Work out the finished part from the listing and answer in its coordinate system (mm). A direction names the side the tool comes from. Round coordinates to 2 decimals unless told otherwise and drop trailing zeros. Write each loop counter-clockwise with the first axis right and the second up, starting at its lowest first coordinate (ties: lowest second). Pieces come first, ordered by that corner, then holes. Notation, with made-up numbers: (-29.5, -38.75) - (25.5, -38.75) arc R32 ccw to (25.5, -3.75) - close; hole circle Ø1 at (-6, 57). An arc over 180 degrees is marked (long way). Answer as a JSON object with one key per item and string values.
```python
from build123d import *

# Parameters (mm, degrees)
BOSS_EXTRUDE1_DEPTH = 33
BOSS_EXTRUDE2_DEPTH = 33
FILLET1_R           = 4
FILLET3_R           = 4
SKETCH3_R           = 1.35
CUT_EXTRUDE1_DEPTH  = 10
SKETCH4_R           = 2.5
CUT_EXTRUDE2_DEPTH  = 1
FILLET4_R           = 4


with BuildPart() as part:
    # Sketch1 → Boss-Extrude1 (new body)
    with BuildSketch(Plane.XY):
        with BuildLine():
            Line((-9.736529156, -5.734980384), (-6, -5.734980384))
            ThreePointArc((-6, -5.734980384), (0, 8.3), (6, -5.734980384))
            Line((6, -5.734980384), (9.736529156, -5.734980384))
            ThreePointArc((9.736529156, -5.734980384), (0, 11.3), (-9.736529156, -5.734980384))
        make_face()
    extrude(amount=BOSS_EXTRUDE1_DEPTH)

    # Sketch2 → Boss-Extrude2 (add)
    with BuildSketch(Plane(origin=(0, 0, 0), x_dir=(-1, 0, 0), z_dir=(0, 0, -1))):
        with BuildLine():
            Line((-10.464206022, 4.265019616), (-18.736529156, 4.265019616))
            Line((-18.736529156, 4.265019616), (-18.736529156, -10.734980384))
            Line((-18.736529156, -10.734980384), (-38.736529156, -10.734980384))
            Line((-38.736529156, -10.734980384), (-38.736529156, -13.734980384))
            Line((-38.736529156, -13.734980384), (-13.736529156, -13.734980384))
            Line((-13.736529156, -13.734980384), (-13.736529156, -5.734980384))
            Line((-13.736529156, -5.734980384), (-9.736529156, -5.734980384))
            ThreePointArc((-9.736529156, -5.734980384), (-11.270200772, -0.820106438), (-10.464206022, 4.265019616))
        make_face()
    extrude(amount=-BOSS_EXTRUDE2_DEPTH)

    # Fillet1
    fillet1_edges = [part.edges().sort_by_distance(p)[0] for p in [
        (18.736529156, 4.265019616, 16.5),
        (10.464206022, 4.265019616, 16.5),
    ]]
    fillet(fillet1_edges, radius=FILLET1_R)

    # Fillet3
    fillet3_edges = [part.edges().sort_by_distance(p)[0] for p in [
        (13.736529156, -5.734980384, 16.5),
    ]]
    fillet(fillet3_edges, radius=FILLET3_R)

    # Sketch3 → Cut-Extrude1 (cut)
    with BuildSketch(Plane(origin=(0, -10.734980384, 0), x_dir=(1, 0, 0), z_dir=(0, 1, 0))):
        with Locations(Location((22.736529156, -4.5, 0), (0, 0, 180))):
            Circle(SKETCH3_R)
        with Locations(Location((34.736529156, -4.5, 0), (0, 0, 180))):
            Circle(SKETCH3_R)
        with Locations(Location((34.736529156, -28.5, 0), (0, 0, 180))):
            Circle(SKETCH3_R)
        with Locations(Location((22.736529156, -28.5, 0), (0, 0, 180))):
            Circle(SKETCH3_R)
    extrude(amount=-CUT_EXTRUDE1_DEPTH, mode=Mode.SUBTRACT)

    # Sketch4 → Cut-Extrude2 (cut)
    with BuildSketch(Plane(origin=(0, -10.734980384, 0), x_dir=(1, 0, 0), z_dir=(0, 1, 0))):
        with Locations(Location((22.736529156, -28.5, 0), (0, 0, 180))):
            Circle(SKETCH4_R)
        with Locations(Location((34.736529156, -28.5, 0), (0, 0, 180))):
            Circle(SKETCH4_R)
        with Locations(Location((34.736529156, -4.5, 0), (0, 0, 180))):
            Circle(SKETCH4_R)
        with Locations(Location((22.736529156, -4.5, 0), (0, 0, 180))):
            Circle(SKETCH4_R)
    extrude(amount=-CUT_EXTRUDE2_DEPTH, mode=Mode.SUBTRACT)

    # Fillet4
    fillet4_edges = [part.edges().sort_by_distance(p)[0] for p in [
        (38.736529156, -12.234980384, 0),
        (38.736529156, -12.234980384, 33),
    ]]
    fillet(fillet4_edges, radius=FILLET4_R)


solid = part.part
```
Item 1: Consider line 1 along Y through (x, z) = (19.5, 19); line 2 along X through (y, z) = (-3.25, 12); line 3 along X through (y, z) = (-11.5, 6). Determine where each line is inside the solid, lowest interval first.
Results found:
{"line 1": "-13.73 to -10.73", "line 2": "-10.82 to -7.64, 7.64 to 18.74", "line 3": "13.74 to 20.74, 24.74 to 32.74, 36.74 to 38.74"}
Item 2: For faces 1 (the cylindrical face through (20.35, -11.23, 5.25)), 2 (the flat face through (8, -5.735, 16)), 3 (the flat face through (14, 4.265, 16)), determine the directions among +Z, -Z, +X, -X, +Y, -Y from which every point of the face is accessible in a straight line to the end or side of a thin tool.
Results found:
{"face 1": "+Y", "face 2": "+Z, -Z, -X, -Y", "face 3": "+Z, -Z, +X, +Y"}
Item 3: Determine the mould class of faces 4 (the flat face through (22, -11.735, 27)), 5 (the cylindrical face through (37.534, -12.256, 1.141)), 6 (the flat face through (10, -1, 33)) for opening direction X: pulls with the +X half, pulls with the -X half, needs draft (parallel to the pull), parting line crosses it, or undercut.
Results found:
{"face 4": "undercut", "face 5": "pulls with the +X half", "face 6": "needs draft"}
Item 4: A cutting plane is placed at C-C (y = 10). Write down the section's boundary in (x, z).
Results found:
{"outline": "(-5.26, 0) - (5.26, 0) - (5.26, 33) - (-5.26, 33) - close"}
Item 5: Each of these flat-tipped pins is pushed along its axis until it touches: P1, Ø12, axis at y = -7, z = 19.5, coming from the -X side; P2, Ø5, axis at x = -5, z = 11.5, coming from the +Y side; P3, Ø3, axis at x = 22.74, z = 4.5, coming from the +Y side (3 decimals); P4, Ø10, axis at x = 0, y = 0, coming from the +Z side. Where does it stop, or does it pass through?
Results found:
{"P1": "x = -11.26", "P2": "y = 11.02", "P3": "y = -11.735", "P4": "through"}
Item 6: A cutting plane is placed at A-A (z = 21). Write down the section's boundary in (x, y).
Results found:
{"outline": "(-9.74, -5.73) - (-6, -5.73) arc R8.3 cw (long way) to (6, -5.73) - (9.74, -5.73) arc R4 cw to (13.74, -9.73) - (13.74, -13.73) - (38.74, -13.73) - (38.74, -10.73) - (18.74, -10.73) - (18.74, 0.27) arc R4 ccw to (14.74, 4.27) - (12.88, 4.27) arc R4 cw to (9.51, 6.1) arc R11.3 ccw to start"}
Item 7: A cutting plane is placed at B-B (x = 0). Write down the section's boundary in (y, z).
Results found:
{"outline": "(8.3, 0) - (11.3, 0) - (11.3, 33) - (8.3, 33) - close"}
